from build123d import *

# Parameters (mm, degrees)
BOSS_EXTRUDE1_DEPTH      = 82
SKETCH5_R                = 10
CUT_EXTRUDE1_DEPTH       = 12
CUT_EXTRUDE2_REACH       = 156.211
SKETCH6_R                = 9
CUT_EXTRUDE4_REACH       = 152.745
SKETCH8_R                = 26
CUT_EXTRUDE5_REACH       = 157.769
FILLET3_R                = 41
SKETCH13_R               = 39
CUT_EXTRUDE6_DEPTH       = 2.5
M4_CLEARANCE_HOLE1_D     = 4.5
M4_CLEARANCE_HOLE1_DEPTH = 7.5
FILLET5_R                = 0.8
CHAMFER2_SIZE            = 5
BOSS_EXTRUDE3_START      = -82
BOSS_EXTRUDE3_DEPTH      = 82
SKETCH19_R               = 39
CUT_EXTRUDE7_DEPTH       = 20
FILLET6_START            = -82.0000001
FILLET6_DEPTH            = 82.0000001
FILLET6_START_2          = -26
FILLET6_2_DEPTH          = 52


with BuildPart() as part:
    # Sketch1 → Boss-Extrude1 (new body)
    with BuildSketch(Plane.XY):
        Polygon((0, 0), (-72, 0), (-82, 0), (-82, 104), (-72, 104), (-72, 10), (-15, 10), (-15, 74), (0, 74), align=None)
    extrude(amount=-BOSS_EXTRUDE1_DEPTH)

    # Sketch5 → Cut-Extrude1 (cut)
    with BuildSketch(Plane.ZY.offset(15)):
        with Locations(Location((-41, 58, 0), (0, 0, 270))):
            Circle(SKETCH5_R)
    extrude(amount=-CUT_EXTRUDE1_DEPTH, mode=Mode.SUBTRACT)

    # Sketch6 → Cut-Extrude2 (cut, up to next)
    with BuildSketch(Plane.ZY.offset(3), mode=Mode.PRIVATE) as cut_extrude2_sk1:
        with Locations(Location((-41, 58, 0), (0, 0, 270))):
            Circle(SKETCH6_R)
    cut_extrude2_tool1 = extrude(cut_extrude2_sk1.sketch, amount=-CUT_EXTRUDE2_REACH, mode=Mode.PRIVATE) & part.part
    add(cut_extrude2_tool1.solids().sort_by_distance((-3, 58, -41))[0], mode=Mode.SUBTRACT)

    # Sketch8 → Cut-Extrude4 (cut, up to next)
    with BuildSketch(Plane(origin=(-72, 0, 0), x_dir=(0, 0, -1), z_dir=(1, 0, 0)), mode=Mode.PRIVATE) as cut_extrude4_sk1:
        with Locations(Location((41, 58, 0), (0, 0, 90))):
            Circle(SKETCH8_R)
    cut_extrude4_tool1 = extrude(cut_extrude4_sk1.sketch, amount=-CUT_EXTRUDE4_REACH, mode=Mode.PRIVATE) & part.part
    add(cut_extrude4_tool1.solids().sort_by_distance((-72, 58, -41))[0], mode=Mode.SUBTRACT)

    # Sketch10 → Cut-Extrude5 (cut, up to next)
    with BuildSketch(Plane(origin=(0, 0, 0), x_dir=(0, 0, -1), z_dir=(1, 0, 0)), mode=Mode.PRIVATE) as cut_extrude5_sk1:
        with BuildLine():
            Line((0, 74), (0, 16))
            Line((0, 16), (11.714285714, 19.492525222))
            ThreePointArc((11.714285714, 19.492525222), (22.035674515, 26.706536079), (26, 38.658822172))
            Line((26, 38.658822172), (26, 59))
            ThreePointArc((26, 59), (30.393398282, 69.606601718), (41, 74))
            Line((41, 74), (0, 74))
        make_face()
    cut_extrude5_tool1 = extrude(cut_extrude5_sk1.sketch, amount=-CUT_EXTRUDE5_REACH, mode=Mode.PRIVATE) & part.part
    # Sketch10 → Cut-Extrude5 (cut, up to next)
    with BuildSketch(Plane(origin=(0, 0, 0), x_dir=(0, 0, -1), z_dir=(1, 0, 0)), mode=Mode.PRIVATE) as cut_extrude5_sk2:
        with BuildLine():
            Line((82, 74), (41, 74))
            ThreePointArc((41, 74), (51.606601718, 69.606601718), (56, 59))
            Line((56, 59), (56, 38.658822172))
            ThreePointArc((56, 38.658822172), (59.964325485, 26.706536079), (70.285714286, 19.492525222))
            Line((70.285714286, 19.492525222), (82, 16))
            Line((82, 16), (82, 74))
        make_face()
    cut_extrude5_tool2 = extrude(cut_extrude5_sk2.sketch, amount=-CUT_EXTRUDE5_REACH, mode=Mode.PRIVATE) & part.part
    add(cut_extrude5_tool1.solids().sort_by_distance((0, 48.321716, -12.955067))[0], mode=Mode.SUBTRACT)
    add(cut_extrude5_tool2.solids().sort_by_distance((0, 48.321716, -69.044933))[0], mode=Mode.SUBTRACT)

    # Fillet3
    fillet3_edges = [part.edges().sort_by_distance(p)[0] for p in [
        (-77, 104, -82),
        (-77, 104, 0),
    ]]
    fillet(fillet3_edges, radius=FILLET3_R - 0.0001)  # a hair under: the kernel refuses the full size

    # Sketch13 → Cut-Extrude6 (cut)
    with BuildSketch(Plane.ZY.offset(82)):
        with Locations((-41, 58)):
            Circle(SKETCH13_R)
    extrude(amount=-CUT_EXTRUDE6_DEPTH, mode=Mode.SUBTRACT)

    # M4 Clearance Hole1
    with Locations(Plane.ZY.offset(79.5)):
        with Locations((-41, 90), (-9, 58), (-41, 26), (-73, 58)):
            Hole(M4_CLEARANCE_HOLE1_D / 2, depth=M4_CLEARANCE_HOLE1_DEPTH)

    # Fillet5
    fillet5_edges = [part.edges().sort_by_distance(p)[0] for p in [
        (-3, 68, -41),
    ]]
    fillet(fillet5_edges, radius=FILLET5_R)

    # Mirror1: part across plane


with BuildPart() as part_1:
    add(part.part)
    add(part.part.mirror(Plane(origin=(0, 74, -82), x_dir=(0, 0, 1), z_dir=(1, 0, 0))))

    # Chamfer2
    chamfer2_edges = [part_1.edges().sort_by_distance(p)[0] for p in [
        (72, 10, -41),
        (-72, 10, -41),
    ]]
    chamfer(chamfer2_edges, length=CHAMFER2_SIZE)

    # Sketch18 → Boss-Extrude3 (add)
    with BuildSketch(Plane.XY.offset(BOSS_EXTRUDE3_START)):
        with BuildLine():
            Line((-72, 35), (-68.226174588, 23))
            ThreePointArc((-68.226174588, 23), (-64.602862357, 17.937742252), (-58.686782574, 16))
            Line((-58.686782574, 16), (0, 16))
            Line((0, 16), (0, 10))
            Line((0, 10), (-67, 10))
            Line((-67, 10), (-72, 15))
            Line((-72, 15), (-72, 35))
        make_face()
    boss_extrude3 = extrude(amount=BOSS_EXTRUDE3_DEPTH)

    # Mirror2: Boss-Extrude3 across plane
    add(boss_extrude3.mirror(Plane(origin=(0, 0, 0), x_dir=(0, 0, 1), z_dir=(1, 0, 0))))

    # Sketch19 → Cut-Extrude7 (cut)
    with BuildSketch(Plane(origin=(-72, 0, 0), x_dir=(0, 0, -1), z_dir=(1, 0, 0))):
        with Locations(Location((41, 58, 0), (0, 0, 180))):
            Circle(SKETCH19_R)
    cut_extrude7 = extrude(amount=CUT_EXTRUDE7_DEPTH, mode=Mode.SUBTRACT)

    # Mirror3: Cut-Extrude7 across plane
    add(cut_extrude7.mirror(Plane(origin=(0, 0, 0), x_dir=(0, 0, 1), z_dir=(1, 0, 0))), mode=Mode.SUBTRACT)

    # Fillet6: read off the stored shape, not the designer's step
    # Fillet6 outline → Fillet6 (add)
    with BuildSketch(Plane.XY.offset(FILLET6_START)):
        with BuildLine():
            Line((15, 16), (25, 16))
            ThreePointArc((25, 16), (17.928932188, 18.928932188), (15, 26))
            Line((15, 26), (15, 16))
        make_face()
        with BuildLine():
            ThreePointArc((-15, 26), (-17.928932188, 18.928932188), (-25, 16))
            Line((-25, 16), (-15, 16))
            Line((-15, 16), (-15, 26))
        make_face()
    extrude(amount=FILLET6_DEPTH)

    # Fillet6 2 outline → Fillet6 2 (cut)
    with BuildSketch(Plane.YZ.offset(FILLET6_START_2)):
        with BuildLine():
            Line((19.492525222, -70.285714286), (16, -82))
            Line((16, -82), (26, -82.0000001))
            Line((26, -82.0000001), (26, -60.516001123))
            ThreePointArc((26, -60.516001123), (22.013361061, -64.912681821), (19.492525222, -70.285714286))
        make_face()
        with BuildLine():
            Line((26, 0), (16, 0))
            Line((16, 0), (19.492525222, -11.714285714))
            ThreePointArc((19.492525222, -11.714285714), (22.013361061, -17.087318179), (26, -21.483998877))
            Line((26, -21.483998877), (26, 0))
        make_face()
    extrude(amount=FILLET6_2_DEPTH, mode=Mode.SUBTRACT)


solid = part_1.part
Part model, mm, in its own coordinate system. A direction names the side the tool comes from. Give positions to 0.01 mm unless a question says otherwise; leave off trailing zeros. Order: outer loops, then holes, each group sorted by start corner. A loop starts at its lowest first (then second) coordinate and runs counter-clockwise, first axis right, second up. Notation, with made-up numbers: (26.25, -21) - (53.25, -21) arc R21 ccw to (53.25, -15) - close; hole circle Ø1 at (18.5, 20.5). An arc over 180 degrees is marked (long way). Use a Markdown table: item, result.
1) Probe L1, parallel to X at y = 31, z = -42.5; L2, parallel to Y at x = -74, z = -41; L3, parallel to Y at x = 74.5, z = -39. List the from-to ranges inside material, lowest first. Write a range as from..to.
Checked values:
| item | result |
|---|---|
| L1 | -79.5..-72, -15..15, 72..79.5 |
| L2 | 0..23.75, 28.25..32, 84..87.75, 92.25..104 |
| L3 | 0..24.97, 27.03..32.08, 83.92..88.97, 91.03..103.95 |
2) Saw through at C-C on x = -21.5. List the corners of the cut face in (y, z), plus the area to 3 significant figures.
Checked values:
| item | result |
|---|---|
| outline | (0, -82) - (16, -82) - (16.63, -79.88) - (16.63, -2.12) - (16, 0) - (0, 0) - close |
| area | 1,360 mm² |
3) 3-axis set-ups, long thin cutter, end or side, ignore diameter. For faces 4 (the cylindrical face through (-64.674, 17.99, -41.574)), 5 (the flat face through (-0.35, 17.77, -76.06)), 6 (the flat face through (-0.35, 17.722, -5.775)), 7 (the cylindrical face through (75.697, 23.804, -40.512)): which of +Z, -Z, +X, -X, +Y, -Y reach the whole face in a straight line?
Checked values:
| item | result |
|---|---|
| face 4 | +Z, -Z, +Y |
| face 5 | -Z, +Y |
| face 6 | +Z, +Y |
| face 7 | +X |
4) Two-plate mould, pull along X, no slides. Class faces 1 (the cylindrical face through (75.697, 87.804, -40.512)), 2 (the cylindrical face through (-69.643, 19.003, -40.487)), 3 (the flat face through (-79.5, 85, -42)): +X half, -X half, draft (parallel to the pull), parting line (faces both ways), or undercut.
Checked values:
| item | result |
|---|---|
| face 1 | draft |
| face 2 | undercut |
| face 3 | -X half |
5) Saw through at A-A on y = 90. List the corners of the cut face in (x, z), plus the area to 3 significant figures.
Checked values:
| item | result |
|---|---|
| outline | (-82, -71.85) - (-72, -71.85) - (-72, -43.25) - (-79.5, -43.25) - (-79.5, -63.29) - (-82, -63.29) - close; (-82, -18.71) - (-79.5, -18.71) - (-79.5, -38.75) - (-72, -38.75) - (-72, -10.15) - (-82, -10.15) - close; (72, -71.85) - (82, -71.85) - (82, -63.29) - (79.5, -63.29) - (79.5, -43.25) - (72, -43.25) - close; (72, -38.75) - (79.5, -38.75) - (79.5, -18.71) - (82, -18.71) - (82, -10.15) - (72, -10.15) - close |
| area | 944 mm² |
6) Flat gauge pins, fed straight in: P1, Ø5, axis at y = 26, z = -41, coming from the -X side; P2, Ø7, axis at y = 26, z = -41, coming from the +X side; P3, Ø10, axis at x = -48, z = -19.5, coming from the +Y side; P4, Ø4, axis at y = 58, z = -73, coming from the +X side. Where does each tip first touch, or does it go through?
Checked values:
| item | result |
|---|---|
| P1 | x = -79.5 |
| P2 | x = 79.5 |
| P3 | y = 16 |
| P4 | through |
7) Saw through at B-B on y = 72. List the corners of the cut face in (x, z), plus the area to 3 significant figures.
Checked values:
| item | result |
|---|---|
| outline | (-82, -81) - (-72, -81) - (-72, -62.91) - (-79.5, -62.91) - (-79.5, -77.4) - (-82, -77.4) - close; (-82, -4.6) - (-79.5, -4.6) - (-79.5, -19.09) - (-72, -19.09) - (-72, -1) - (-82, -1) - close; (-15, -48.48) - (15, -48.48) - (15, -33.52) - (-15, -33.52) - close; (72, -81) - (82, -81) - (82, -77.4) - (79.5, -77.4) - (79.5, -62.91) - (72, -62.91) - close; (72, -19.09) - (79.5, -19.09) - (79.5, -4.6) - (82, -4.6) - (82, -1) - (72, -1) - close |
| area | 1,030 mm² |
